Work out the finished part from the listing and answer in its coordinate system (mm). Face numbers are marked on the shaded views. Round coordinates to 2 decimals unless told otherwise and drop trailing zeros. Loops run counter-clockwise (first coordinate to the right, second up) from the corner with the lowest first, then second, coordinate; pieces in that order, holes last. Notation, with made-up numbers: (1.5, -21.5) - (7.5, -21.5) arc R11 ccw to (7.5, -7.5) - close; hole circle Ø2 at (3, -35.5). An arc over 180 degrees is marked (long way). Answer as CSV lines item,"result". Start each with the question number.
Q1. Section D-D on x = 11 is taken. Write down the section's boundary in (y, z), then the cut area to 3 significant figures.
Q2. Section B-B on z = -0.25 is taken. Write down the section's boundary in (x, y).
Q3. The mould has two halves that part along X. Classify the marked faces 1, 2 and 3: +X half, -X half, draft (parallel to the pull), parting line (faces both ways), or undercut.
Q4. Straight lines are drawn through the part: L1, parallel to X at y = 7.25, z = 0; L2, parallel to X at y = -1.5, z = -1; L3, parallel to Z at x = -7.5, y = -0.75. For each, find the intervals that lie inside material, in ascending order. Write a range as [from, to].
Q5. Section C-C on x = 0 is taken. Write down the section's boundary in (y, z), then the cut area to 3 significant figures.
Q6. Section A-A on y = 2 is taken. Write down the section's boundary in (x, z).
Q7. Each of these flat-tipped pins is pushed along its axis until it touches: pin 1 Ø8 at (x, y) = (11.5, -7) entering from +Z; pin 2 Ø1 at (x, y) = (1.5, -7) entering from -Z; pin 3 Ø6 at (x, y) = (-8.5, 8) entering from +Z; pin 4 Ø4 at (x, z) = (0, -1.54) entering from -Y. Where does it stop, or does it pass through?
```python
from build123d import *

# Parameters (mm, degrees)
SKETCH1_R           = 2.6
BOSS_EXTRUDE1_DEPTH = 12.5


with BuildPart() as part:
    # Sketch1 → Boss-Extrude1 (new, symmetric)
    with BuildSketch(Plane(origin=(0, 0, 0), x_dir=(1, 0, 0), z_dir=(0, 1, 0))):
        with BuildLine():
            Line((18.269584171, -2.356974332), (20.210940503, 2.329874452))
            ThreePointArc((20.210940503, 2.329874452), (20.19858704, 2.544220241), (20.022938795, 2.667688533))
            ThreePointArc((20.022938795, 2.667688533), (0.438109454, 4.261682942), (-19.146719886, 2.667688533))
            ThreePointArc((-19.146719886, 2.667688533), (-19.322368131, 2.544220241), (-19.334721594, 2.329874452))
            Line((-19.334721594, 2.329874452), (-17.393365262, -2.356974332))
            ThreePointArc((-17.393365262, -2.356974332), (-17.286501727, -2.477513642), (-17.128021481, -2.506384946))
            ThreePointArc((-17.128021481, -2.506384946), (0.438109454, -1.164961325), (18.00424039, -2.506384946))
            ThreePointArc((18.00424039, -2.506384946), (18.162720636, -2.477513642), (18.269584171, -2.356974332))
        make_face()
        with Locations(Location((0, 1.536674283, 0), (0, 0, 270))):
            Circle(SKETCH1_R, mode=Mode.SUBTRACT)
    extrude(amount=BOSS_EXTRUDE1_DEPTH, both=True)


solid = part.part
```
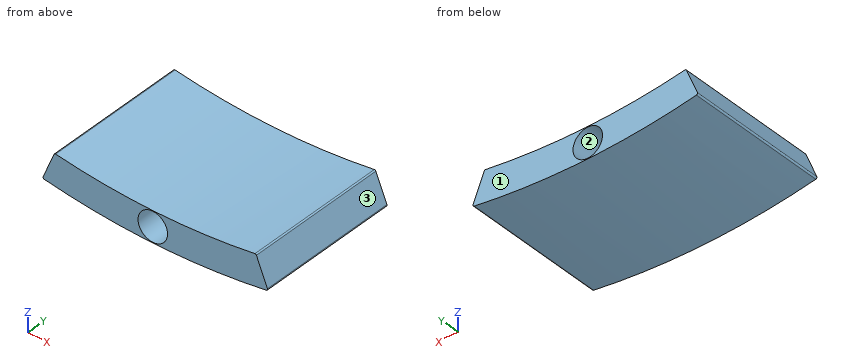
Findings:
1,outline,"(-12.5, -3.8) - (12.5, -3.8) - (12.5, 1.65) - (-12.5, 1.65) - close"
1,area,"136 mm^2"
2,outline,"(-18.47, -12.5) - (-2.26, -12.5) - (-2.26, 12.5) - (-18.47, 12.5) - close; (2.26, -12.5) - (19.35, -12.5) - (19.35, 12.5) - (2.26, 12.5) - close"
3,face 1,"draft"
3,face 2,"undercut"
3,face 3,"+X half"
4,L1,"x = [-18.37, -2.1], [2.1, 19.25]"
4,L2,"x = [-18.78, -2.54], [2.54, 19.66]"
4,L3,"z = [-4, 1.44]"
5,outline,"(-12.5, -4.26) - (12.5, -4.26) - (12.5, -4.14) - (-12.5, -4.14) - close; (-12.5, 1.06) - (12.5, 1.06) - (12.5, 1.17) - (-12.5, 1.17) - close"
5,area,"5.67 mm^2"
6,outline,"(-19.33, -2.33) arc R0.25 ccw to (-19.15, -2.67) arc R121.11 ccw to (20.02, -2.67) arc R0.25 ccw to (20.21, -2.33) - (18.27, 2.36) arc R0.25 ccw to (18, 2.51) arc R115.69 cw to (-17.13, 2.51) arc R0.25 ccw to (-17.39, 2.36) - close; hole circle Ø5.2 at (0, -1.54)"
7,pin 1,"stops at z = 2.15"
7,pin 2,"stops at z = -4.26"
7,pin 3,"stops at z = 1.78"
7,pin 4,"passes through"
